Design review of the part built by this model. Coordinates are the model's own, in mm. Face numbers are marked on the shaded views. A direction names the side the tool comes from. Coordinates: 2 decimals unless noted, no trailing zeros. Write each loop counter-clockwise with the first axis right and the second up, starting at its lowest first coordinate (ties: lowest second). Pieces come first, ordered by that corner, then holes. Notation, with made-up numbers: (-9.75, 81) - (13.25, 81) arc R25 ccw to (13.25, 97) - close; hole circle Ø1 at (-1, 32.25). An arc over 180 degrees is marked (long way). One line per item, written item: value.
from build123d import *

# Parameters (mm, degrees)
SKETCH4_R      = 2.031992692
SKETCH4_R_2    = 1.905
EXTRUDE3_DEPTH = 10.8966


with BuildPart() as part:
    # Sketch4 → Extrude3 (new, symmetric)
    with BuildSketch(Plane.XY):
        with BuildLine():
            Line((-42.343481517, -2.990600597), (-42.343481517, 17.964399403))
            ThreePointArc((-42.343481517, 17.964399403), (-41.413545547, 20.209463433), (-39.168481517, 21.139399403))
            Line((-39.168481517, 21.139399403), (-15.038481517, 21.139399403))
            Line((-15.038481517, 21.139399403), (-15.038481517, 18.236569756))
            ThreePointArc((-15.038481517, 18.236569756), (-14.108545547, 15.991505726), (-11.863481517, 15.061569756))
            Line((-11.863481517, 15.061569756), (9.257081626, 15.061569756))
            ThreePointArc((9.257081626, 15.061569756), (11.502145656, 15.991505726), (12.432081626, 18.236569756))
            Line((12.432081626, 18.236569756), (12.432081626, 22.681569756))
            Line((12.432081626, 22.681569756), (52.437081626, 22.681569756))
            ThreePointArc((52.437081626, 22.681569756), (54.682145656, 21.751633786), (55.612081626, 19.506569756))
            Line((55.612081626, 19.506569756), (55.612081626, -9.945714332))
            ThreePointArc((55.612081626, -9.945714332), (56.542017596, -12.190778362), (58.787081626, -13.120714332))
            Line((58.787081626, -13.120714332), (61.618454053, -13.120714332))
            Line((61.618454053, -13.120714332), (61.618454053, -19.76149571))
            Line((61.618454053, -19.76149571), (12.432081626, -19.76149571))
            Line((12.432081626, -19.76149571), (12.432081626, -17.323430244))
            ThreePointArc((12.432081626, -17.323430244), (11.502145656, -15.078366214), (9.257081626, -14.148430244))
            Line((9.257081626, -14.148430244), (-18.530518374, -14.148430244))
            ThreePointArc((-18.530518374, -14.148430244), (-20.775582404, -15.078366214), (-21.705518374, -17.323430244))
            Line((-21.705518374, -17.323430244), (-21.705518374, -19.76149571))
            Line((-21.705518374, -19.76149571), (-40.618560355, -19.76149571))
            Line((-40.618560355, -19.76149571), (-40.618560355, -13.120714332))
            Line((-40.618560355, -13.120714332), (-35.040518374, -13.120714332))
            ThreePointArc((-35.040518374, -13.120714332), (-32.795454344, -12.190778362), (-31.865518374, -9.945714332))
            Line((-31.865518374, -9.945714332), (-31.865518374, -9.340600597))
            ThreePointArc((-31.865518374, -9.340600597), (-32.795454344, -7.095536567), (-35.040518374, -6.165600597))
            Line((-35.040518374, -6.165600597), (-39.168481517, -6.165600597))
            ThreePointArc((-39.168481517, -6.165600597), (-41.413545547, -5.235664628), (-42.343481517, -2.990600597))
        make_face()
        with Locations((-27.221195322, -14.622613425)):
            Circle(SKETCH4_R, mode=Mode.SUBTRACT)
        with Locations((52.287415303, -15.678066597)):
            Circle(SKETCH4_R_2, mode=Mode.SUBTRACT)
        with Locations((13.846294556, -12.683763681)):
            Circle(SKETCH4_R_2, mode=Mode.SUBTRACT)
        with Locations((13.846294556, 13.596903192)):
            Circle(SKETCH4_R_2, mode=Mode.SUBTRACT)
        with Locations((-37.474326825, 16.270244711)):
            Circle(SKETCH4_R_2, mode=Mode.SUBTRACT)
        with Locations((-16.452694446, 13.596903192)):
            Circle(SKETCH4_R_2, mode=Mode.SUBTRACT)
        with Locations((50.814973838, 17.884461968)):
            Circle(SKETCH4_R_2, mode=Mode.SUBTRACT)
        with BuildLine():
            Line((49.262081626, -12.243430244), (49.262081626, 13.156569756))
            ThreePointArc((49.262081626, 13.156569756), (48.332145656, 15.401633786), (46.087081626, 16.331569756))
            Line((46.087081626, 16.331569756), (20.687081626, 16.331569756))
            ThreePointArc((20.687081626, 16.331569756), (18.442017596, 15.401633786), (17.512081626, 13.156569756))
            Line((17.512081626, 13.156569756), (17.512081626, 9.981569756))
            Line((17.512081626, 9.981569756), (-20.118481517, 9.981569756))
            Line((-20.118481517, 9.981569756), (-20.118481517, 11.614399403))
            ThreePointArc((-20.118481517, 11.614399403), (-21.048417487, 13.859463433), (-23.293481517, 14.789399403))
            Line((-23.293481517, 14.789399403), (-32.818481517, 14.789399403))
            ThreePointArc((-32.818481517, 14.789399403), (-35.063545547, 13.859463433), (-35.993481517, 11.614399403))
            Line((-35.993481517, 11.614399403), (-35.993481517, 2.089399403))
            ThreePointArc((-35.993481517, 2.089399403), (-35.063545547, -0.155664628), (-32.818481517, -1.085600597))
            Line((-32.818481517, -1.085600597), (-26.785518374, -1.085600597))
            Line((-26.785518374, -1.085600597), (-26.785518374, -5.893430244))
            ThreePointArc((-26.785518374, -5.893430244), (-25.855582404, -8.138494274), (-23.610518374, -9.068430244))
            Line((-23.610518374, -9.068430244), (17.512081626, -9.068430244))
            Line((17.512081626, -9.068430244), (17.512081626, -12.243430244))
            ThreePointArc((17.512081626, -12.243430244), (18.442017596, -14.488494274), (20.687081626, -15.418430244))
            Line((20.687081626, -15.418430244), (46.087081626, -15.418430244))
            ThreePointArc((46.087081626, -15.418430244), (48.332145656, -14.488494274), (49.262081626, -12.243430244))
        make_face(mode=Mode.SUBTRACT)
    extrude(amount=EXTRUDE3_DEPTH, both=True)


solid = part.part
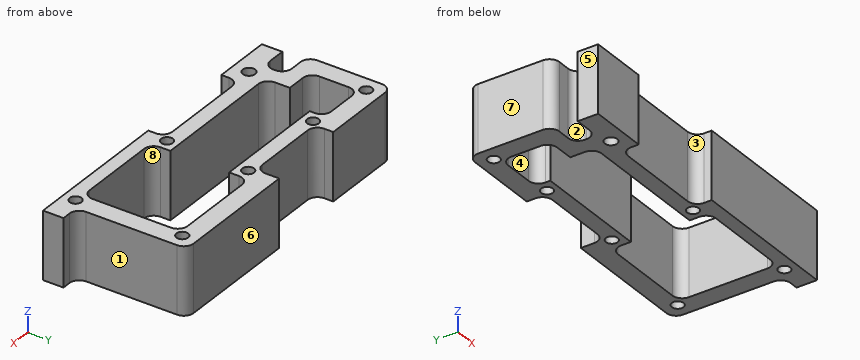
1. Wall thickness on line 1 along Y through (x, z) = (8.5, -8.75); line 2 along X through (y, z) = (-15, -5); line 3 along X through (y, z) = (11, 6.5): over which ranges is each line inside the solid? List them lowest first.
Answer block:
line 1: y = -14.15 to -9.07, 9.98 to 15.06
line 2: x = -40.62 to -29.22, -25.22 to -20.69, 11.42 to 19.11, 47.66 to 50.51, 54.07 to 61.62
line 3: x = -42.34 to -35.99, -20.12 to 17.51, 49.26 to 55.61
2. Consider section C-C, the plane z = -9. Give the number of separate pieces and of enclosed holes in the cut face, then the cut area to 3 significant figures.
Answer block:
separate pieces: 1
enclosed holes: 8
area: 1,580 mm^2
3. Consider section B-B, the plane x = 4.5. Write out the cut boundary in (y, z).
Answer block:
outline: (-14.15, -10.9) - (-9.07, -10.9) - (-9.07, 10.9) - (-14.15, 10.9) - close; (9.98, -10.9) - (15.06, -10.9) - (15.06, 10.9) - (9.98, 10.9) - close
4. For the marked faces 1, 2, 3, 4 and 5, list the 3-axis set-ups (+Z, -Z, +X, -X, +Y, -Y) from which the entire face can be reached by the end or side of a thin tool; tool diameter is ignored.
Answer block:
face 1: +Z, -Z, +X, +Y
face 2: +Z, -Z, -X
face 3: +Z, -Z, -Y
face 4: +Z, -Z
face 5: +Z, -Z, -X, -Y
5. Mouldability with a two-part tool opening along X and no side actions: class the marked faces 6, 7 and 8 as released by +X, released by -X, zero draft, split by the parting line, or undercut.
Answer block:
face 6: zero draft
face 7: released by -X
face 8: undercut
6. Consider section A-A, the plane x = 22.5. Write out the cut boundary in (y, z).
Answer block:
outline: (-19.76, -10.9) - (-15.42, -10.9) - (-15.42, 10.9) - (-19.76, 10.9) - close; (16.33, -10.9) - (22.68, -10.9) - (22.68, 10.9) - (16.33, 10.9) - close
7. Insertion check: pin 1 Ø3.5 at (y, z) = (-10, -4) entering from +X; pin 2 Ø1.5 at (y, z) = (-14, -3) entering from -X; pin 3 Ø5.5 at (y, z) = (-4.5, 5) entering from +X; pin 4 Ø3.5 at (x, y) = (50.81, 17.88) entering from +Z. Each pin has a flat end and moves straight along its axis. Give the tip position at first contact, or say it passes through.
Answer block:
pin 1: stops at x = 56.17
pin 2: stops at x = -40.62
pin 3: stops at x = 55.61
pin 4: passes through
